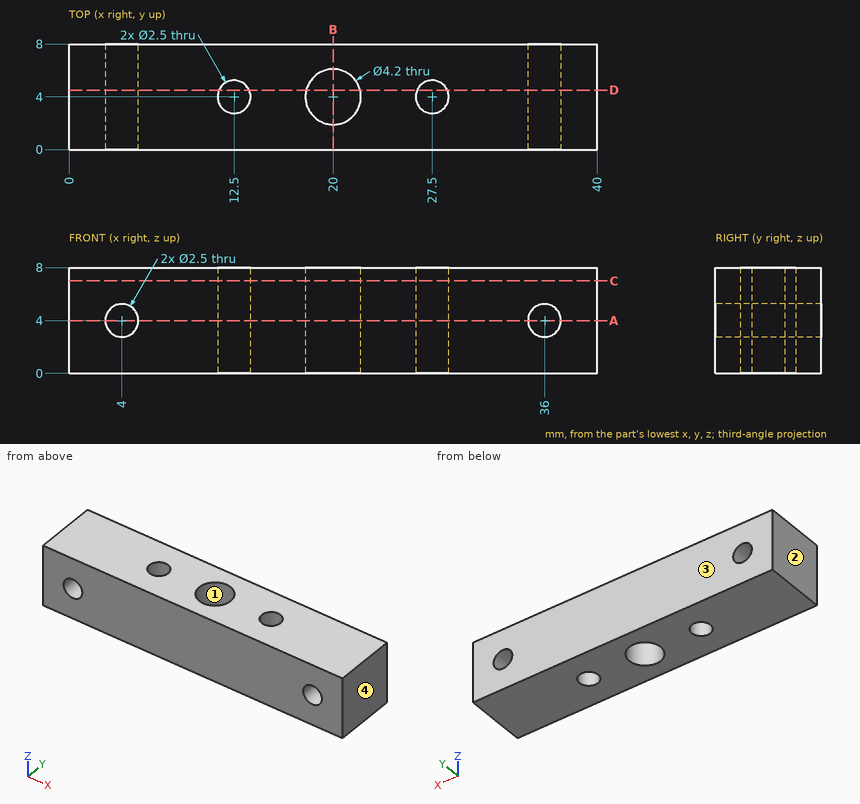
Design review of the part shown in the three views and the two pictorial views. Dimensions are in mm from the part's minimum x, y and z. Give positions to 0.01 mm unless a question says otherwise; leave off trailing zeros. Loops run counter-clockwise (first coordinate to the right, second up) from the corner with the lowest first, then second, coordinate; pieces in that order, holes last. Notation, with made-up numbers: M 88.5,5 L 109.5,5 A7 cw 109.5,18 Z; hole C 60.25,-32 d10. An arc over 180 degrees is marked long. Answer as a JSON object with one key per item and string values.
Item 1: Wall thickness on line 1 along Y through (x, z) = (20, 2.75); line 2 along X through (y, z) = (3.75, 2); line 3 along Y through (x, z) = (27.5, 2.5): over which ranges is each line inside the solid? List them lowest first.
Output values:
{"line 1": "y = 0 to 1.9, 6.1 to 8", "line 2": "x = 0 to 11.28, 13.72 to 17.91, 22.09 to 26.28, 28.72 to 40", "line 3": "y = 0 to 2.75, 5.25 to 8"}
Item 2: We need section C-C (z = 7). State the section outline as (x, y) points, and give its area (3 significant figures).
Output values:
{"outline": "M 0,0 L 40,0 L 40,8 L 0,8 Z; hole C 12.5,4 d2.5; hole C 20,4 d4.2; hole C 27.5,4 d2.5", "area": "296 mm2"}
Item 3: We need section D-D (y = 4.5). State the section outline as (x, z) points, and give its area (3 significant figures).
Output values:
{"outline": "M 0,0 L 11.35,0 L 11.35,8 L 0,8 Z; M 13.65,0 L 17.96,0 L 17.96,8 L 13.65,8 Z; M 22.04,0 L 26.35,0 L 26.35,8 L 22.04,8 Z; M 28.65,0 L 40,0 L 40,8 L 28.65,8 Z; hole C 4,4 d2.5; hole C 36,4 d2.5", "area": "241 mm2"}
Item 4: We need section A-A (z = 4). State the section outline as (x, y) points.
Output values:
{"outline": "M 0,0 L 2.75,0 L 2.75,8 L 0,8 Z; M 5.25,0 L 34.75,0 L 34.75,8 L 5.25,8 Z; M 37.25,0 L 40,0 L 40,8 L 37.25,8 Z; hole C 12.5,4 d2.5; hole C 20,4 d4.2; hole C 27.5,4 d2.5"}
Item 5: Mouldability with a two-part tool opening along X and no side actions: class the marked faces 1, 2, 3 and 4 as pulls with the +X half, pulls with the -X half, needs draft (parallel to the pull), parting line crosses it, or undercut.
Output values:
{"face 1": "undercut", "face 2": "pulls with the -X half", "face 3": "needs draft", "face 4": "pulls with the +X half"}
Item 6: We need section B-B (x = 20). State the section outline as (y, z) points.
Output values:
{"outline": "M 0,0 L 1.9,0 L 1.9,8 L 0,8 Z; M 6.1,0 L 8,0 L 8,8 L 6.1,8 Z"}
